from build123d import *

# Parameters (mm, degrees)
SKETCH1_W           = 43
SKETCH1_H           = 36
SKETCH1_R           = 1.5
BOSS_EXTRUDE1_DEPTH = 2.4
SKETCH2_W           = 12
SKETCH2_H           = 16
BOSS_EXTRUDE2_DEPTH = 11


with BuildPart() as part:
    # Sketch1 → Boss-Extrude1 (new body)
    with BuildSketch(Plane.XY):
        with Locations((21.5, 18)):
            Rectangle(SKETCH1_W, SKETCH1_H)
        with Locations((39, 6)):
            Circle(SKETCH1_R, mode=Mode.SUBTRACT)
        with Locations((4.1, 30.3)):
            Circle(SKETCH1_R, mode=Mode.SUBTRACT)
        with Locations((39.1, 31.4)):
            Circle(SKETCH1_R, mode=Mode.SUBTRACT)
    extrude(amount=BOSS_EXTRUDE1_DEPTH)

    # Sketch2 → Boss-Extrude2 (add)
    with BuildSketch(Plane.XY.offset(2.4)):
        with Locations((11, 4.591861043)):
            Rectangle(SKETCH2_W, SKETCH2_H)
    extrude(amount=BOSS_EXTRUDE2_DEPTH)


solid = part.part
Model file for the job. Use its own axes, mm. A direction names the side the tool comes from. Give positions to 0.01 mm unless a question says otherwise; leave off trailing zeros. Loops run counter-clockwise (first coordinate to the right, second up) from the corner with the lowest first, then second, coordinate; pieces in that order, holes last. Notation, with made-up numbers: (15, 21.5) -> (49, 21.5) arc R31 cw to (49, 45.5) -> close; hole circle Ø8 at (81, 28). An arc over 180 degrees is marked (long way). Use a Markdown table: item, result. Add a question column.
(1) Slice it at D-D on x = 39.1. List the corners of the cut face in (y, z), and give its area (3 significant figures).
(2) Mould opens along X. For faces 6 (the cylindrical face through (37.8, 5.1, 1.2)), 7 (the flat face through (43, 18, 1)), 8 (the flat face through (5, 4, 8)), 9 (the flat face through (11, -2, 2.4)) say: +X half, -X half, draft (parallel to the pull), parting line (faces both ways), or undercut.
(3) Slice it at B-B on y = 6. List the corners of the cut face in (x, z), and give its area (3 significant figures).
(4) Drop flat-ended pins along their axis: pin 1 Ø3.5 at (x, z) = (12, 7) entering from +Y; pin 2 Ø2.5 at (x, z) = (23.5, 1) entering from -Y; pin 3 Ø4 at (x, y) = (38, 10) entering from +Z. Give the stop position or say it passes through.
(5) Slice it at C-C on x = 4.1. List the corners of the cut face in (y, z).
(6) Tool access for faces 1 (the flat face through (17, 4, 8)), 2 (the flat face through (21, 0, 1)), 3 (the flat face through (0, 18, 1)), 4 (the flat face through (21, 36, 1)), 5 (the flat face through (11, 12.592, 8)): list every direction of +Z, -Z, +X, -X, +Y, -Y with a clear straight run to the whole face (end or side of a thin tool).
(7) Wall check: line 1 along Y through (x, z) = (39, 0.7); line 2 along Z through (x, y) = (30, 17.5); line 3 along Y through (x, z) = (15, 0.5). Give the ranges that are in metal, low to high.
(8) Slice it at A-A on z = 1. List the corners of the cut face in (x, y), and give its area (3 significant figures).
Filled sheet:
| question | item | result |
|---|---|---|
| 1 | outline | (0, 0) -> (4.5, 0) -> (4.5, 2.4) -> (0, 2.4) -> close; (7.5, 0) -> (29.9, 0) -> (29.9, 2.4) -> (7.5, 2.4) -> close; (32.9, 0) -> (36, 0) -> (36, 2.4) -> (32.9, 2.4) -> close |
| 1 | area | 72.0 mm2 |
| 2 | face 6 | undercut |
| 2 | face 7 | +X half |
| 2 | face 8 | -X half |
| 2 | face 9 | draft |
| 3 | outline | (0, 0) -> (37.5, 0) -> (37.5, 2.4) -> (17, 2.4) -> (17, 13.4) -> (5, 13.4) -> (5, 2.4) -> (0, 2.4) -> close; (40.5, 0) -> (43, 0) -> (43, 2.4) -> (40.5, 2.4) -> close |
| 3 | area | 228 mm2 |
| 4 | pin 1 | y = 12.59 |
| 4 | pin 2 | y = 0 |
| 4 | pin 3 | z = 2.4 |
| 5 | outline | (0, 0) -> (28.8, 0) -> (28.8, 2.4) -> (0, 2.4) -> close; (31.8, 0) -> (36, 0) -> (36, 2.4) -> (31.8, 2.4) -> close |
| 6 | face 1 | +Z, +X, +Y, -Y |
| 6 | face 2 | -Z, +X, -X, -Y |
| 6 | face 3 | +Z, -Z, -X, +Y, -Y |
| 6 | face 4 | +Z, -Z, +X, -X, +Y |
| 6 | face 5 | +Z, +X, -X, +Y |
| 7 | line 1 | 0 to 4.5, 7.5 to 29.9, 32.9 to 36 |
| 7 | line 2 | 0 to 2.4 |
| 7 | line 3 | 0 to 36 |
| 8 | outline | (0, 0) -> (43, 0) -> (43, 36) -> (0, 36) -> close; hole circle Ø3 at (4.1, 30.3); hole circle Ø3 at (39, 6); hole circle Ø3 at (39.1, 31.4) |
| 8 | area | 1,530 mm2 |
